from build123d import *

# Parameters (mm, degrees)
F0_R     = 2.55
F0_W     = 27.4615384615
F0_H     = 34
F1_DEPTH = 6
F2_R     = 2.55
F3_DEPTH = 6
F5_DEPTH = 6.001
F6_R     = 5


with BuildPart() as f1:
    # F0 (on Top) → F1 (new body)
    with BuildSketch(Plane.XY):
        with BuildLine():
            Line((26.5, 39), (-26.5, 39))
            ThreePointArc((-26.5, 39), (-30.0355339059, 37.5355339059), (-31.5, 34))
            Line((-31.5, 34), (-31.5, -34))
            ThreePointArc((-31.5, -34), (-30.0355339059, -37.5355339059), (-26.5, -39))
            Line((-26.5, -39), (26.5, -39))
            ThreePointArc((26.5, -39), (30.0355339059, -37.5355339059), (31.5, -34))
            Line((31.5, -34), (31.5, 34))
            ThreePointArc((31.5, 34), (30.0355339059, 37.5355339059), (26.5, 39))
        make_face()
        with Locations((-26, -33.5)):
            Circle(F0_R, mode=Mode.SUBTRACT)
        with Locations((26, -33.5)):
            Circle(F0_R, mode=Mode.SUBTRACT)
        Rectangle(F0_W, F0_H, mode=Mode.SUBTRACT)
        with Locations((-26, 33.5)):
            Circle(F0_R, mode=Mode.SUBTRACT)
        with Locations((26, 33.5)):
            Circle(F0_R, mode=Mode.SUBTRACT)
    extrude(amount=F1_DEPTH)

    # F2 (on Top) → F3 (join, through all)
    with BuildSketch(Plane.XY):
        with BuildLine():
            Line((-44.8330235429, 18.5), (44.8330235429, 18.5))
            ThreePointArc((44.8330235429, 18.5), (0, 48.5), (-44.8330235429, 18.5))
        make_face()
        with Locations((-26, 33.5)):
            Circle(F2_R, mode=Mode.SUBTRACT)
        with Locations((26, 33.5)):
            Circle(F2_R, mode=Mode.SUBTRACT)
    extrude(amount=F3_DEPTH)

    # F4 (on Top) → F5 (cut, through all)
    with BuildSketch(Plane.XY):
        with BuildLine():
            Line((13.7307692308, 17), (13.7307692308, 35.96826346))
            ThreePointArc((13.7307692308, 35.96826346), (0, 38.5), (-13.7307692308, 35.96826346))
            Line((-13.7307692308, 35.96826346), (-13.7307692308, 17))
            Line((-13.7307692308, 17), (13.7307692308, 17))
        make_face()
    extrude(amount=F5_DEPTH, mode=Mode.SUBTRACT)

    # F6
    f6_edges = [f1.edges().sort_by_distance(p)[0] for p in [
        (44.833024, 18.5, 3),
        (-31.5, 18.5, 3),
        (31.5, 18.5, 3),
        (13.730769, 35.968263, 3),
        (-13.730769, 35.968263, 3),
        (-44.833024, 18.5, 3),
    ]]
    fillet(f6_edges, radius=F6_R)


solid = f1.part
Geometry check sheet. Reference: the model listing, model coordinates, mm. A direction names the side the tool comes from. Give positions to 0.01 mm unless a question says otherwise; leave off trailing zeros. Loops run counter-clockwise (first coordinate to the right, second up) from the corner with the lowest first, then second, coordinate; pieces in that order, holes last. Notation, with made-up numbers: M 69.5,33 L 81.5,33 A29 cw 81.5,57 Z; hole C 29.25,42 d6. An arc over 180 degrees is marked long. Write each question's results on one line, items separated by ' | '.
1) Thickness scan on line 1 (Y direction, x = -26, z = 1.8); line 2 (X direction, y = -16, z = 0.35); line 3 (Y direction, x = 0, z = 4.85). Record the ranges inside material, lowest first.
Answers follow:
line 1: -39 to -36.05, -30.95 to 30.95, 36.05 to 40.94 | line 2: -31.5 to -13.73, 13.73 to 31.5 | line 3: -39 to -17, 38.5 to 48.5
2) Release check for a two-part mould opening along X. For faces 4 (the face through (-13.731, 7, 3)), 5 (the face through (0, -39, 3)), 6 (the face through (-27.9, 35.2, 3)), 7 (the face through (31.5, -11, 3)) record: +X half, -X half, draft (parallel to the pull), parting line (faces both ways), or undercut.
Answers follow:
face 4: undercut | face 5: draft | face 6: undercut | face 7: +X half
3) Section check D-D, the plane y = -24.5. Record the boundary of the cut face in (x, z).
Answers follow:
outline: M -31.5,0 L 31.5,0 L 31.5,6 L -31.5,6 Z
4) Gauge pin test, flat ends, axial feed: pin 1 (1.5 mm diameter, centred on x = 18.5, z = 1, fed in from +Y); pin 2 (3 mm diameter, centred on x = -3.5, z = 2.5, fed in from +Y); pin 3 (1.8 mm diameter, centred on y = 0.5, z = 3, fed in from +X). Record the tip position at first contact, or that the pin passes through.
Answers follow:
pin 1: y = 45.14 | pin 2: y = 48.46 | pin 3: x = 31.5
5) Tool access check on faces 1 (the face through (30, -37.57, 2.96)), 2 (the face through (0.1, 38.5, 3)), 3 (the face through (-31.5, -10, 3)). Record the directions out of +Z, -Z, +X, -X, +Y, -Y that give a thin tool (end or side, any length) a straight path to the whole face; none if there is none.
Answers follow:
face 1: +Z, -Z, +X, -Y | face 2: +Z, -Z | face 3: +Z, -Z, -X, -Y
6) Section check C-C, the plane y = 33.5. Record the boundary of the cut face in (x, z), plus the area to 3 significant figures.
Answers follow:
outline: M -35.07,0 L -28.55,0 L -28.55,6 L -35.07,6 Z; M -23.45,0 L -13.59,0 L -13.59,6 L -23.45,6 Z; M 13.59,0 L 23.45,0 L 23.45,6 L 13.59,6 Z; M 28.55,0 L 35.07,0 L 35.07,6 L 28.55,6 Z | area: 197 mm2
7) Section check B-B, the plane z = 1.6. Record the boundary of the cut face in (x, y).
Answers follow:
outline: M -40.81,26.2 A5 ccw -36.61,18.5 L -36.5,18.5 A5 cw -31.5,13.5 L -31.5,-34 A5 ccw -26.5,-39 L 26.5,-39 A5 ccw 31.5,-34 L 31.5,13.5 A5 cw 36.5,18.5 L 36.61,18.5 A5 ccw 40.81,26.2 A48.5 ccw Z; hole C -26,-33.5 d5.1; hole C -26,33.5 d5.1; hole M -13.73,-17 L 13.73,-17 L 13.73,32.34 A5 ccw 10.03,37.17 A38.5 ccw -10.03,37.17 A5 ccw -13.73,32.34 Z; hole C 26,-33.5 d5.1; hole C 26,33.5 d5.1
8) Section check A-A, the plane y = -0.5. Record the boundary of the cut face in (x, z).
Answers follow:
outline: M -31.5,0 L -13.73,0 L -13.73,6 L -31.5,6 Z; M 13.73,0 L 31.5,0 L 31.5,6 L 13.73,6 Z
